Can you work these out from the model? Positions are in its coordinate system, mm. Coordinates: 2 decimals unless noted, no trailing zeros. Loops run counter-clockwise (first coordinate to the right, second up) from the corner with the lowest first, then second, coordinate; pieces in that order, holes last.
```python
from build123d import *

# Parameters (mm, degrees)
SKETCH1_W            = 50
SKETCH1_H            = 9.1
BOSS_EXTRUDE1_DEPTH  = 2
SKETCH2_W            = 25
SKETCH2_H            = 6.6
CUT_EXTRUDE1_DEPTH   = 2
SKETCH3_R            = 1.8
CUT_EXTRUDE2_DEPTH   = 2
SKETCH4_W            = 66.4
SKETCH4_H            = 130
BOSS_EXTRUDE2_DEPTH  = 2
SKETCH5_W            = 66.4
SKETCH5_H            = 2
BOSS_EXTRUDE3_DEPTH  = 2.5
SKETCH6_W            = 8.6
SKETCH6_H            = 62.5
BOSS_EXTRUDE4_DEPTH  = 2
SKETCH7_R            = 1.8
SKETCH7_W            = 3
SKETCH7_H            = 5
CUT_EXTRUDE3_DEPTH   = 2
SKETCH8_W            = 25
SKETCH8_H            = 45
CUT_EXTRUDE4_DEPTH   = 20
SKETCH9_W            = 25
SKETCH9_H            = 10
BOSS_EXTRUDE5_DEPTH  = 2
SKETCH10_W           = 34.7
SKETCH10_H           = 27.07
BOSS_EXTRUDE6_DEPTH  = 2
SKETCH11_R           = 1.8
CUT_EXTRUDE5_DEPTH   = 2
SKETCH12_R           = 1.8
CUT_EXTRUDE6_DEPTH   = 2
SKETCH13_W           = 2
SKETCH13_H           = 2
BOSS_EXTRUDE7_DEPTH  = 44
SKETCH14_W           = 2
SKETCH14_H           = 2
BOSS_EXTRUDE8_DEPTH  = 46
BOSS_EXTRUDE9_DEPTH  = 2
SKETCH16_W           = 42
SKETCH16_H           = 43
BOSS_EXTRUDE10_DEPTH = 2
SKETCH18_R           = 1.8
CUT_EXTRUDE7_DEPTH   = 2
BOSS_EXTRUDE11_DEPTH = 2
BOSS_EXTRUDE12_DEPTH = 2
SKETCH21_W           = 2
SKETCH21_H           = 2
BOSS_EXTRUDE13_DEPTH = 10
SKETCH22_W           = 62.5
SKETCH22_H           = 2
BOSS_EXTRUDE14_DEPTH = 2
SKETCH23_W           = 62.5
SKETCH23_H           = 2
BOSS_EXTRUDE15_DEPTH = 2
SKETCH25_W           = 3
SKETCH25_H           = 5
CUT_EXTRUDE8_DEPTH   = 10


with BuildPart() as part:
    # Sketch1 → Boss-Extrude1 (new body)
    with BuildSketch(Plane(origin=(0, 0, 0), x_dir=(1, 0, 0), z_dir=(0, 1, 0))):
        with Locations((25, 4.55)):
            Rectangle(SKETCH1_W, SKETCH1_H)
    extrude(amount=BOSS_EXTRUDE1_DEPTH)

    # Sketch2 → Cut-Extrude1 (cut)
    with BuildSketch(Plane(origin=(0, 2, 0), x_dir=(1, 0, 0), z_dir=(0, 1, 0))):
        with Locations((25, 5.8)):
            Rectangle(SKETCH2_W, SKETCH2_H)
    extrude(amount=-CUT_EXTRUDE1_DEPTH, mode=Mode.SUBTRACT)

    # Sketch3 → Cut-Extrude2 (cut)
    with BuildSketch(Plane(origin=(0, 2, 0), x_dir=(1, 0, 0), z_dir=(0, 1, 0))):
        with Locations(Location((6.25, 5.8, 0), (0, 0, 270))):
            Circle(SKETCH3_R)
        with Locations(Location((43.75, 5.8, 0), (0, 0, 270))):
            Circle(SKETCH3_R)
    extrude(amount=-CUT_EXTRUDE2_DEPTH, mode=Mode.SUBTRACT)

    # Sketch4 → Boss-Extrude2 (add)
    with BuildSketch(Plane(origin=(0, 2, 0), x_dir=(1, 0, 0), z_dir=(0, 1, 0))):
        with Locations((25, -65)):
            Rectangle(SKETCH4_W, SKETCH4_H)
    extrude(amount=-BOSS_EXTRUDE2_DEPTH)

    # Sketch5 → Boss-Extrude3 (add)
    with BuildSketch(Plane.XY.offset(130)):
        with Locations((25, 1)):
            Rectangle(SKETCH5_W, SKETCH5_H)
    extrude(amount=BOSS_EXTRUDE3_DEPTH)

    # Sketch6 → Boss-Extrude4 (add)
    with BuildSketch(Plane(origin=(0, 2, 0), x_dir=(1, 0, 0), z_dir=(0, 1, 0))):
        with Locations((-12.5, -101.25)):
            Rectangle(SKETCH6_W, SKETCH6_H)
        with Locations((62.5, -101.25)):
            Rectangle(SKETCH6_W, SKETCH6_H)
    extrude(amount=-BOSS_EXTRUDE4_DEPTH)

    # Sketch7 → Cut-Extrude3 (cut)
    with BuildSketch(Plane(origin=(0, 2, 0), x_dir=(1, 0, 0), z_dir=(0, 1, 0))):
        with Locations(Location((-13.5, -77, 0), (0, 0, 270))):
            Circle(SKETCH7_R)
        with Locations(Location((-13.5, -101.25, 0), (0, 0, 270))):
            Circle(SKETCH7_R)
        with Locations(Location((-13.5, -125.5, 0), (0, 0, 270))):
            Circle(SKETCH7_R)
        with Locations(Location((63.5, -77, 0), (0, 0, 270))):
            Circle(SKETCH7_R)
        with Locations(Location((63.5, -101.25, 0), (0, 0, 270))):
            Circle(SKETCH7_R)
        with Locations(Location((63.5, -125.5, 0), (0, 0, 270))):
            Circle(SKETCH7_R)
        with Locations((-13.5, -117.5)):
            Rectangle(SKETCH7_W, SKETCH7_H)
        with Locations((63.5, -117.5)):
            Rectangle(SKETCH7_W, SKETCH7_H)
    extrude(amount=-CUT_EXTRUDE3_DEPTH, mode=Mode.SUBTRACT)

    # Sketch8 → Cut-Extrude4 (cut)
    with BuildSketch(Plane(origin=(0, 2, 0), x_dir=(1, 0, 0), z_dir=(0, 1, 0))):
        with Locations((25, -22.5)):
            Rectangle(SKETCH8_W, SKETCH8_H)
    extrude(amount=-CUT_EXTRUDE4_DEPTH, mode=Mode.SUBTRACT)

    # Sketch9 → Boss-Extrude5 (add)
    with BuildSketch(Plane(origin=(0, 2, 0), x_dir=(1, 0, 0), z_dir=(0, 1, 0))):
        with Locations((25, -5)):
            Rectangle(SKETCH9_W, SKETCH9_H)
    extrude(amount=-BOSS_EXTRUDE5_DEPTH)

    # Sketch10 → Boss-Extrude6 (add)
    with BuildSketch(Plane(origin=(0, 2, 0), x_dir=(1, 0, 0), z_dir=(0, 1, 0))):
        with Locations((-25.55, -29.535)):
            Rectangle(SKETCH10_W, SKETCH10_H)
        with Locations((75.55, -29.535)):
            Rectangle(SKETCH10_W, SKETCH10_H)
    extrude(amount=-BOSS_EXTRUDE6_DEPTH)

    # Sketch11 → Cut-Extrude5 (cut)
    with BuildSketch(Plane(origin=(0, 2, 0), x_dir=(1, 0, 0), z_dir=(0, 1, 0))):
        with Locations(Location((-36.9, -19.25, 0), (0, 0, 270))):
            Circle(SKETCH11_R)
        with Locations(Location((-36.9, -39.82, 0), (0, 0, 270))):
            Circle(SKETCH11_R)
        with Locations(Location((-22.6, -19.25, 0), (0, 0, 270))):
            Circle(SKETCH11_R)
        with Locations(Location((-22.6, -39.82, 0), (0, 0, 270))):
            Circle(SKETCH11_R)
    extrude(amount=-CUT_EXTRUDE5_DEPTH, mode=Mode.SUBTRACT)

    # Sketch12 → Cut-Extrude6 (cut)
    with BuildSketch(Plane(origin=(0, 2, 0), x_dir=(1, 0, 0), z_dir=(0, 1, 0))):
        with Locations(Location((72.6, -19.25, 0), (0, 0, 270))):
            Circle(SKETCH12_R)
        with Locations(Location((86.9, -19.25, 0), (0, 0, 270))):
            Circle(SKETCH12_R)
        with Locations(Location((72.6, -39.82, 0), (0, 0, 270))):
            Circle(SKETCH12_R)
        with Locations(Location((86.9, -39.82, 0), (0, 0, 270))):
            Circle(SKETCH12_R)
    extrude(amount=-CUT_EXTRUDE6_DEPTH, mode=Mode.SUBTRACT)

    # Sketch13 → Boss-Extrude7 (add)
    with BuildSketch(Plane.ZY.offset(42.9)):
        with Locations((15, 1)):
            Rectangle(SKETCH13_W, SKETCH13_H)
        with Locations((44.07, 1)):
            Rectangle(SKETCH13_W, SKETCH13_H)
    extrude(amount=-BOSS_EXTRUDE7_DEPTH)

    # Sketch14 → Boss-Extrude8 (add)
    with BuildSketch(Plane(origin=(92.9, 0, 0), x_dir=(0, 0, -1), z_dir=(1, 0, 0))):
        with Locations((-15, 1)):
            Rectangle(SKETCH14_W, SKETCH14_H)
        with Locations((-44.07, 1)):
            Rectangle(SKETCH14_W, SKETCH14_H)
    extrude(amount=-BOSS_EXTRUDE8_DEPTH)

    # Sketch15 → Boss-Extrude9 (add)
    with BuildSketch(Plane(origin=(0, 2, 0), x_dir=(1, 0, 0), z_dir=(0, 1, 0))):
        with BuildLine():
            Line((-8.2, -14), (-8.2, -8))
            ThreePointArc((-8.2, -8), (-9.957359313, -12.242640687), (-14.2, -14))
            Line((-14.2, -14), (-8.2, -14))
        make_face()
        with BuildLine():
            Line((-14.2, -45.07), (-8.2, -45.07))
            Line((-8.2, -45.07), (-8.2, -51.07))
            ThreePointArc((-8.2, -51.07), (-9.957359313, -46.827359313), (-14.2, -45.07))
        make_face()
        with BuildLine():
            ThreePointArc((64.2, -45.07), (59.957359313, -46.827359313), (58.2, -51.07))
            Line((58.2, -51.07), (58.2, -45.07))
            Line((58.2, -45.07), (64.2, -45.07))
        make_face()
        with BuildLine():
            ThreePointArc((58.2, -8), (59.957359313, -12.242640687), (64.2, -14))
            Line((64.2, -14), (58.2, -14))
            Line((58.2, -14), (58.2, -8))
        make_face()
    extrude(amount=-BOSS_EXTRUDE9_DEPTH)

    # Sketch16 → Boss-Extrude10 (add)
    with BuildSketch(Plane(origin=(0, 2, 0), x_dir=(1, 0, 0), z_dir=(0, 1, 0))):
        with Locations((25, -154)):
            Rectangle(SKETCH16_W, SKETCH16_H)
    extrude(amount=-BOSS_EXTRUDE10_DEPTH)

    # Sketch18 → Cut-Extrude7 (cut)
    with BuildSketch(Plane(origin=(0, 2, 0), x_dir=(1, 0, 0), z_dir=(0, 1, 0))):
        with Locations(Location((8.74, -171.03, 0), (0, 0, 270))):
            Circle(SKETCH18_R)
        with Locations(Location((41.26, -171.03, 0), (0, 0, 270))):
            Circle(SKETCH18_R)
        with Locations(Location((8.74, -138.5, 0), (0, 0, 270))):
            Circle(SKETCH18_R)
        with Locations(Location((41.26, -138.5, 0), (0, 0, 270))):
            Circle(SKETCH18_R)
    extrude(amount=-CUT_EXTRUDE7_DEPTH, mode=Mode.SUBTRACT)

    # Sketch19 → Boss-Extrude11 (add)
    with BuildSketch(Plane(origin=(0, 2, 0), x_dir=(1, 0, 0), z_dir=(0, 1, 0))):
        with BuildLine():
            ThreePointArc((-16.8, -70), (-10.718881682, -67.481118318), (-8.2, -61.4))
            Line((-8.2, -61.4), (-8.2, -70))
            Line((-8.2, -70), (-16.8, -70))
        make_face()
        with BuildLine():
            ThreePointArc((58.2, -61.4), (60.718881682, -67.481118318), (66.8, -70))
            Line((66.8, -70), (58.2, -70))
            Line((58.2, -70), (58.2, -61.4))
        make_face()
    extrude(amount=-BOSS_EXTRUDE11_DEPTH)

    # Sketch20 → Boss-Extrude12 (add)
    with BuildSketch(Plane(origin=(0, 2, 0), x_dir=(1, 0, 0), z_dir=(0, 1, 0))):
        with BuildLine():
            Line((-2, -132.5), (4, -132.5))
            Line((4, -132.5), (4, -138.5))
            ThreePointArc((4, -138.5), (2.242640687, -134.257359313), (-2, -132.5))
        make_face()
        with BuildLine():
            ThreePointArc((52, -132.5), (47.757359313, -134.257359313), (46, -138.5))
            Line((46, -138.5), (46, -132.5))
            Line((46, -132.5), (52, -132.5))
        make_face()
    extrude(amount=-BOSS_EXTRUDE12_DEPTH)

    # Sketch21 → Boss-Extrude13 (add)
    with BuildSketch(Plane(origin=(0, 0, -9.1), x_dir=(-1, 0, 0), z_dir=(0, 0, -1))):
        with Locations((-51, 1)):
            Rectangle(SKETCH21_W, SKETCH21_H)
        with Locations((-36.5, 1)):
            Rectangle(SKETCH21_W, SKETCH21_H)
        with Locations((-13.5, 1)):
            Rectangle(SKETCH21_W, SKETCH21_H)
        with Locations((1, 1)):
            Rectangle(SKETCH21_W, SKETCH21_H)
    extrude(amount=-BOSS_EXTRUDE13_DEPTH)

    # Sketch22 → Boss-Extrude14 (add)
    with BuildSketch(Plane.ZY.offset(16.8)):
        with Locations((101.25, 1)):
            Rectangle(SKETCH22_W, SKETCH22_H)
    extrude(amount=BOSS_EXTRUDE14_DEPTH)

    # Sketch23 → Boss-Extrude15 (add)
    with BuildSketch(Plane(origin=(66.8, 0, 0), x_dir=(0, 0, -1), z_dir=(1, 0, 0))):
        with Locations((-101.25, 1)):
            Rectangle(SKETCH23_W, SKETCH23_H)
    extrude(amount=BOSS_EXTRUDE15_DEPTH)

    # Sketch25 → Cut-Extrude8 (cut)
    with BuildSketch(Plane(origin=(0, 2, 0), x_dir=(1, 0, 0), z_dir=(0, 1, 0))):
        with Locations((-11.7, -22.5)):
            Rectangle(SKETCH25_W, SKETCH25_H)
        with Locations((-11.7, -36.57)):
            Rectangle(SKETCH25_W, SKETCH25_H)
        with Locations((61.7, -22.5)):
            Rectangle(SKETCH25_W, SKETCH25_H)
        with Locations((61.7, -36.57)):
            Rectangle(SKETCH25_W, SKETCH25_H)
    extrude(amount=-CUT_EXTRUDE8_DEPTH, mode=Mode.SUBTRACT)


solid = part.part
```
Item 1: Suppose I cut it at B-B, the plane x = -29.5. Please give me the cut outline in (y, z), plus the area to 3 significant figures.
Results are:
outline: (0, 14) - (2, 14) - (2, 45.07) - (0, 45.07) - close
area: 62.1 mm2
Item 2: Suppose I cut it at C-C, the plane z = 89. Please give me the cut outline in (x, y).
Results are:
outline: (-18.8, 0) - (68.8, 0) - (68.8, 2) - (-18.8, 2) - close
Item 3: I need wall thicknesses on line 1 along X through (y, z) = (0.95, 39.82); line 2 along Z through (x, y) = (86.9, 1.65); line 3 along X through (y, z) = (0.55, 101). Which ranges of each line are inside material? Lowest first, please.
Results are:
line 1: x = -42.9 to -38.7, -35.1 to -24.4, -20.8 to 12.5, 37.5 to 70.8, 74.4 to 85.1, 88.7 to 92.9
line 2: z = 14 to 17.45, 21.05 to 38.02, 41.62 to 45.07
line 3: x = -18.8 to -15.28, -11.72 to 61.72, 65.28 to 68.8
Item 4: Suppose I cut it at A-A, the plane y = 0.6. Count the separate pieces of the cut face and the enclosed holes in it, plus the area to 3 significant figures.
Results are:
separate pieces: 1
enclosed holes: 27
area: 13,300 mm2
Item 5: I'm going to push flat-ended pins straight in: P1, Ø1, axis at x = 61, y = 1.5, coming from the -Z side; P2, Ø0.6, axis at y = 1, z = 116.5, coming from the -X side; P3, Ø0.6, axis at y = 1, z = -7, coming from the -X side. Where does each tip first touch, or does it pass through?
Results are:
P1: stops at z = 12.72
P2: stops at x = -18.8
P3: stops at x = -2
Item 6: We'd pull the mould along Z, two halves only. Please class faces 1 (the face through (-10.79, 1.01, 67.55)), 2 (the face through (-35.115, 1.014, 19.016)), 3 (the face through (24, 2, 64)), 4 (the face through (47.804, 1.014, 134.211)): +Z half, -Z half, draft (parallel to the pull), parting line (faces both ways), or undercut.
Results are:
face 1: undercut
face 2: undercut
face 3: draft
face 4: +Z half
